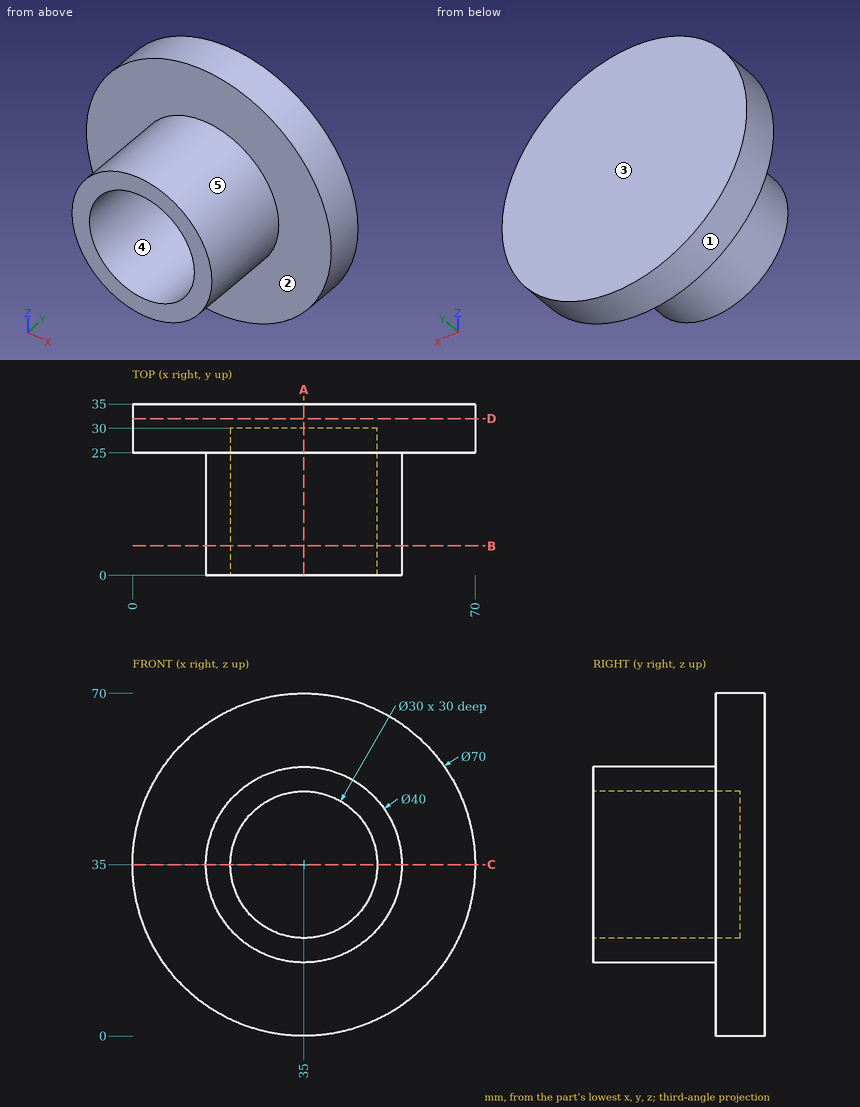
The drawing under review shows one solid part. Ordinate dimensions are in mm from its lowest x, y, z. A direction names the side the tool comes from. Coordinates: 2 decimals unless noted, no trailing zeros. Write each loop counter-clockwise with the first axis right and the second up, starting at its lowest first coordinate (ties: lowest second). Pieces come first, ordered by that corner, then holes. Notation, with made-up numbers: M -23.75,31 L -10.75,31 A23 cw -10.75,54 Z; hole C -38.75,18.5 d11. An arc over 180 degrees is marked long. Put each result on its own line as item: value.
1) Add section C-C on z = 35. Give the boundary of the cut face in (x, y).
Computed:
outline: M 0,25 L 15,25 L 15,0 L 20,0 L 20,30 L 50,30 L 50,0 L 55,0 L 55,25 L 70,25 L 70,35 L 0,35 Z
2) For the marked faces 1 and 2, list the 3-axis set-ups (+Z, -Z, +X, -X, +Y, -Y) from which the entire face can be reached by the end or side of a thin tool; tool diameter is ignored.
Computed:
face 1: +Y, -Y
face 2: -Y
3) Add section B-B on y = 6. Give the boundary of the cut face in (x, z).
Computed:
outline: C 35,35 d40; hole C 35,35 d30
4) Wall thickness on probe 1 along X at (y, z) = (22.5, 35); probe 2 along Z at (x, y) = (35, 26): over which ranges is each line inside the solid? List them lowest first. Write a range as [from, to].
Computed:
probe 1: x = [15, 20], [50, 55]
probe 2: z = [0, 20], [50, 70]
5) Clearance check with flat-ended pins moving along their axes: pin 1 Ø5 at (x, y) = (47, 10.5) entering from -Z; pin 2 Ø10 at (x, y) = (39.5, 9) entering from -Z; pin 3 Ø10 at (x, y) = (27.5, 21.5) entering from +Z. State where each tip first meets the part, or that it passes through.
Computed:
pin 1: stops at z = 17.4
pin 2: stops at z = 15
pin 3: stops at z = 69.78
6) Add section A-A on x = 35. Give the boundary of the cut face in (y, z), then the cut area to 3 significant figures.
Computed:
outline: M 0,15 L 25,15 L 25,0 L 35,0 L 35,70 L 25,70 L 25,55 L 0,55 L 0,50 L 30,50 L 30,20 L 0,20 Z
area: 800 mm2
7) Draft analysis for pull direction Z (two halves, no side actions). For the marked faces 3, 4 and 5, state which applies: released by +Z, released by -Z, zero draft, split by the parting line, or undercut.
Computed:
face 3: zero draft
face 4: undercut
face 5: split by the parting line
8) Add section D-D on y = 32. Give the boundary of the cut face in (x, z).
Computed:
outline: C 35,35 d70
